from build123d import *

# Parameters (mm, degrees)
F0_R          = 50
F1_DEPTH      = 10
F3_DEPTH      = 10
F5_DEPTH      = 10
F5_DEPTH_BACK = 30
F7_R          = 2.5
F8_DEPTH      = 10


with BuildPart() as f1:
    # F0 (on Top) → F1 (new body)
    with BuildSketch(Plane.XY):
        Circle(F0_R)
    extrude(amount=F1_DEPTH)

    # F2 (on face) → F3 (join)
    with BuildSketch(Plane.XY.offset(10)):
        with BuildLine():
            ThreePointArc((-30, 12.5), (-6.373774392, -31.86887196), (32.5, 0))
            ThreePointArc((32.5, 0), (31.86887196, 6.373774392), (30, 12.5))
            ThreePointArc((30, 12.5), (0, 1.418320568), (-30, 12.5))
        make_face()
    extrude(amount=F3_DEPTH)

    # F4 (on face) → F5 (join, two sides)
    with BuildSketch(Plane.XY.offset(20)) as f5_sk:
        with BuildLine():
            ThreePointArc((-0.4808877088, 1.4208261722), (0, 1.418320568), (0.4808877088, 1.4208261722))
            ThreePointArc((0.4808877088, 1.4208261722), (0, 1.5), (-0.4808877088, 1.4208261722))
        make_face()
        with BuildLine():
            ThreePointArc((-0.4808877088, 1.4208261722), (-0.8742620994, -1.2188789036), (1.5, 0))
            ThreePointArc((1.5, 0), (1.2188789036, 0.8742620994), (0.4808877088, 1.4208261722))
            ThreePointArc((0.4808877088, 1.4208261722), (0, 1.418320568), (-0.4808877088, 1.4208261722))
        make_face()
    extrude(amount=F5_DEPTH)
    extrude(f5_sk.sketch, amount=-F5_DEPTH_BACK)

    # F7 (on face) → F8 (join)
    with BuildSketch(Plane.XY.offset(10)):
        with Locations((0, 45.2338345349)):
            Circle(F7_R)
    extrude(amount=F8_DEPTH)


solid = f1.part
Build history of the part. All positions in model axes, mm. A direction names the side the tool comes from. Coordinates: 2 decimals unless noted, no trailing zeros. Order: outer loops, then holes, each group sorted by start corner. A loop starts at its lowest first (then second) coordinate and runs counter-clockwise, first axis right, second up. Notation, with made-up numbers: (71, -13) - (129, -13) arc R14 cw to (129, -3) - close; hole circle Ø6 at (-21, 86.5). An arc over 180 degrees is marked (long way). Write each question's results on one line, items separated by ' | '. Start each with the question number.
Item 1: Band-saw the part on D-D on x = 37. Write the cut outline in (y, z).
Item 2: Band-saw the part on C-C on y = -35. Write the cut outline in (x, z).
Item 3: Flat gauge pins, fed straight in: pin 1 (2 mm diameter, centred on x = -33, y = -13, fed in from +Z); pin 2 (10 mm diameter, centred on x = -16, z = 5, fed in from -Y) (3 decimals); pin 3 (13.5 mm diameter, centred on x = -12, y = -8.5, fed in from +Z); pin 4 (5 mm diameter, centred on x = -15.5, z = 24.5, fed in from +Y). Where does each tip first touch, or does it go through?
Item 4: Wall check: probe 1 along Z at (x, y) = (-40, 25.5); probe 2 along Z at (x, y) = (-16, -12); probe 3 along X at (y, z) = (0, -5). Give the ranges that are in metal, low to high. Write a range as [from, to].
Item 5: Tool access for faces 4 (the face through (0, 45, 20)), 5 (the face through (-1, 12, 10)), 6 (the face through (0, 0, 30)): list every direction of +Z, -Z, +X, -X, +Y, -Y with a clear straight run to the whole face (end or side of a thin tool).
Item 6: Band-saw the part on B-B on y = -8.5. Write the cut outline in (x, z).
Item 7: Band-saw the part on A-A on x = -20. Write the cut outline in (y, z).
Item 8: Mould opens along X. For faces 1 (the face through (-16, 4.28, 14.93)), 2 (the face through (-1, -10, 0)), 3 (the face through (47.69, 15.02, 4.93)) say: released by +X, released by -X, zero draft, split by the parting line, or undercut.
Numbers:
1) outline: (-33.63, 0) - (33.63, 0) - (33.63, 10) - (-33.63, 10) - close
2) outline: (-35.71, 0) - (35.71, 0) - (35.71, 10) - (-35.71, 10) - close
3) pin 1: z = 10 | pin 2: y = -48.775 | pin 3: z = 20 | pin 4: through
4) probe 1: [0, 10] | probe 2: [0, 20] | probe 3: [-1.5, 1.5]
5) face 4: +Z, +X, -X, +Y | face 5: +Z | face 6: +Z, +X, -X, +Y, -Y
6) outline: (-49.27, 0) - (49.27, 0) - (49.27, 10) - (31.37, 10) - (31.37, 20) - (-31.37, 20) - (-31.37, 10) - (-49.27, 10) - close
7) outline: (-45.83, 0) - (45.83, 0) - (45.83, 10) - (5.98, 10) - (5.98, 20) - (-25.62, 20) - (-25.62, 10) - (-45.83, 10) - close
8) face 1: undercut | face 2: zero draft | face 3: split by the parting line
